Autodesk Inventor part; units mm, degrees
ref_plane "YZ Plane" through (0, 0, 0) normal (1, 0, 0) x (0, 1, 0)
ref_plane "XZ Plane" through (0, 0, 0) normal (0, 1, 0) x (-1, 0, 0)
ref_plane "XY Plane" through (0, 0, 0) normal (0, 0, 1) x (1, 0, 0)
sketch "Sketch1" plane through (0, 0, 0) normal (0, 0, 1) x (1, 0, 0)
  line L0 (9.6801, -14.008) -> (7.2052, -11.5331) construction
  line L1 (7.2052, -11.5331) -> (11.5893, -7.1491) construction
  line L2 (11.5893, -7.1491) -> (14.0642, -9.6239) construction
  line L3 (14.0642, -9.6239) -> (9.6801, -14.008) construction
  arc A0 (12.6369, -4.7496) -> (4.7496, -12.6369) centre (0, 0) ccw construction
  line L4 (10.9298, -3.0424) -> (12.6369, -4.7496) construction
  line L5 (11.6618, -4.6122) -> (10.9298, -3.0424) construction
  arc A1 (11.6618, -4.6122) -> (10.8551, -4.47) centre (11.2086, -4.8235) ccw construction
  line L6 (10.7915, -4.5335) -> (10.8551, -4.47) construction
  arc A2 (10.7915, -4.5335) -> (10.6527, -4.9738) centre (11.1451, -4.887) ccw construction
  line L7 (10.915, -6.4612) -> (10.6527, -4.9738) construction
  arc A3 (10.7761, -6.9016) -> (10.915, -6.4612) centre (10.4226, -6.548) ccw construction
  line L8 (6.9016, -10.7761) -> (10.7761, -6.9016) construction
  arc A4 (6.4612, -10.915) -> (6.9016, -10.7761) centre (6.548, -10.4226) ccw construction
  line L9 (6.4612, -10.915) -> (4.9738, -10.6527) construction
  arc A5 (4.9738, -10.6527) -> (4.5335, -10.7915) centre (4.887, -11.1451) ccw construction
  line L10 (4.5335, -10.7915) -> (4.47, -10.8551) construction
  arc A6 (4.47, -10.8551) -> (4.6122, -11.6618) centre (4.8235, -11.2086) ccw construction
  line L11 (4.6122, -11.6618) -> (3.0424, -10.9298) construction
  line L12 (3.0424, -10.9298) -> (4.7496, -12.6369) construction
  line L13 (-1.7167, -14.6498) -> (-1.7167, -17.5) construction
  line L14 (-1.7167, -17.5) -> (1.7167, -17.5) construction
  line L15 (1.7167, -14.6498) -> (1.7167, -17.5) construction
  arc A7 (1.7167, -14.6498) -> (6.9595, -13.0049) centre (0, 0) ccw construction
  arc A8 (6.9595, -13.0049) -> (8.2728, -15.1789) centre (8.2994, -13.6792) ccw construction
  line L16 (8.2728, -15.1789) -> (7.6816, -15.1684) construction
  arc A9 (8.5249, -17.8901) -> (7.6816, -15.1684) centre (7.655, -16.6682) ccw construction
  line L17 (8.5249, -17.8901) -> (13.5161, -14.3366) construction
  line L18 (13.5161, -14.3366) -> (13.5161, -12.2823) construction
  line L19 (13.5161, -12.2823) -> (14.6168, -12.2823) construction
  line L20 (14.6168, -12.2823) -> (14.6168, -1.9776) construction
  arc A10 (14.6168, -1.9776) -> (1.7167, 14.6498) centre (0, 0) ccw construction
  line L21 (1.7167, 14.6498) -> (1.7167, 17.5) construction
  line L22 (-1.7167, 17.5) -> (1.7167, 17.5) construction
  line L23 (-1.7167, 14.6498) -> (-1.7167, 17.5) construction
  arc A11 (-1.7167, 14.6498) -> (-14.2817, -3.6872) centre (0, 0) ccw construction
  line L24 (-14.2817, -3.6872) -> (-15.4135, -5.7935) construction
  arc A12 (-15.4135, -5.7935) -> (-14.5984, -8.502) centre (-13.6517, -6.7402) ccw construction
  line L25 (-14.5984, -8.502) -> (-9.6326, -11.1703) construction
  arc A13 (-9.6326, -11.1703) -> (-1.7167, -14.6498) centre (0, 0) ccw construction
  line L26 (-24.6, 24.6) -> (25.2, -25.2) construction
  line L27 (25.2, 24.6) -> (-24.6, -25.2) construction
  arc A14 (-1.4283, 10.15) -> (-9.5043, -3.8381) centre (0, 0) ccw
  circle A15 centre (0, 0) radius 10.1 construction
  line L28 (-1.4283, 10.15) -> (1.4283, 10.15)
  line L29 (-8.076, -6.3119) -> (-9.5043, -3.8381)
  line L30 (9.5043, -3.8381) -> (8.076, -6.3119)
  arc A16 (1.4283, 10.15) -> (-1.4283, 10.15) centre (0, 0) ccw
  arc A17 (9.5043, -3.8381) -> (1.4283, 10.15) centre (0, 0) ccw
  arc A18 (8.076, -6.3119) -> (9.5043, -3.8381) centre (0, 0) ccw
  arc A19 (-8.076, -6.3119) -> (8.076, -6.3119) centre (0, 0) ccw
  arc A20 (-9.5043, -3.8381) -> (-8.076, -6.3119) centre (0, 0) ccw
  arc A21 (10.7786, -4.5205) -> (10.6704, -4.6789) centre (11.1451, -4.887) ccw construction
  line L31 (10.7786, -4.5205) -> (10.8421, -4.457) construction
  arc A22 (11.7261, -4.7937) -> (10.8421, -4.457) centre (11.2086, -4.8235) ccw construction
  line L32 (11.7261, -4.7937) -> (10.8691, -2.9558) construction
  line L33 (10.8691, -2.9558) -> (12.6297, -4.7164) construction
  line L34 (4.7164, -12.6297) -> (2.9558, -10.8691) construction
  line L35 (2.9558, -10.8691) -> (4.4463, -11.5641) construction
  arc A23 (4.457, -10.8421) -> (4.4463, -11.5641) centre (4.8235, -11.2086) ccw construction
  line L36 (4.457, -10.8421) -> (4.5223, -10.7767) construction
  arc A24 (4.977, -10.6346) -> (4.6789, -10.6704) centre (4.887, -11.1451) ccw
  arc A25 (4.6789, -10.6704) -> (4.5223, -10.7767) centre (4.887, -11.1451) ccw construction
  arc A26 (10.6704, -4.6789) -> (10.6346, -4.977) centre (11.1451, -4.887) ccw
  circle A27 centre (0, 0) radius 12.65
  dimension "d4" = 20.2
  dimension "d5" = 10.15
  dimension "d6" = 20.5
  dimension "d9" = 360
  dimension "d28" = 25.3
extrude "Extrusion1" add sketch "Sketch1" against normal blind 3
sketch "Sketch3" plane through (0, 0, -3) normal (0, 0, -1) x (-1, 0, 0)
  circle A0 centre (0, 0) radius 10.25
  circle A1 centre (0, 0) radius 9
  circle A2 centre (0, 0) radius 11.5312
  circle A3 centre (0, 0) radius 12.65
  dimension "d17" = 18
extrude "Extrusion3" add sketch "Sketch3" along normal blind 10 contours A0 | A2 | A3
sketch "Sketch4" plane through (0, -10.7054, 0) normal (1, 0, 0) x (0, 0, -1)
  line L0 (13, 19.7054) -> (13, 1.7054)
  line L1 (3, 1.7054) -> (3, 19.7054)
  circle A0 centre (11, 10.7054) radius 1.4
  circle A1 centre (5, 10.7054) radius 1.4
  dimension "d24" = 2.8
  dimension "d25" = 2.8
  dimension "d26" = 6
  dimension "d27" = 2
extrude "Extrusion4" cut sketch "Sketch4" against normal through all
properties part number "30_focus_inlet_objective_mount_v7"
Model file for the job. Use its own axes, mm. A direction names the side the tool comes from. Round coordinates to 2 decimals unless told otherwise and drop trailing zeros. Order: outer loops, then holes, each group sorted by start corner. A loop starts at its lowest first (then second) coordinate and runs counter-clockwise, first axis right, second up. Notation, with made-up numbers: (16.5, -9) -> (29.5, -9) arc R19 cw to (29.5, 0) -> close; hole circle Ø7 at (32, 70.5). An arc over 180 degrees is marked (long way). Use one line per item in the form item = value.
Item 1: Cut at B-B, the plane x = 0. Write the cut outline in (y, z).
Returned:
outline = (-12.65, -13) -> (-9, -13) -> (-9, -3) -> (-10.25, -3) -> (-10.25, 0) -> (-12.65, 0) -> close; (9, -13) -> (12.65, -13) -> (12.65, 0) -> (10.25, 0) -> (10.25, -3) -> (9, -3) -> close
Item 2: Drill centre lines: line 1 (Z direction, x = -11.05, y = 0); line 2 (Y direction, x = 0, z = -7.75); line 3 (Z direction, x = 6.5, y = -7.5). Where is each one in solid material? Low to high.
Returned:
line_1 = -13 to -12.4, -9.6 to -6.4, -3.6 to 0
line_2 = -12.65 to -9, 9 to 12.65
line_3 = -13 to -3
Item 3: Cut at D-D, the plane z = -7.75. Write the cut outline in (x, y).
Returned:
outline = circle Ø25.3 at (0, 0); hole circle Ø18 at (0, 0)
Item 4: Cut at A-A, the plane y = 0. Write the cut outline in (x, z).
Returned:
outline = (-12.65, -13) -> (-9, -13) -> (-9, -12.4) -> (-12.65, -12.4) -> close; (-12.65, -9.6) -> (-9, -9.6) -> (-9, -6.4) -> (-12.65, -6.4) -> close; (-12.65, -3.6) -> (-9, -3.6) -> (-9, -3) -> (-10.25, -3) -> (-10.25, 0) -> (-12.65, 0) -> close; (9, -13) -> (12.65, -13) -> (12.65, 0) -> (10.25, 0) -> (10.25, -3) -> (9, -3) -> close
Item 5: Cut at C-C, the plane y = 5.75. Write the cut outline in (x, z).
Returned:
outline = (-11.27, -13) -> (-6.92, -13) -> (-6.92, -3) -> (-8.49, -3) -> (-8.49, 0) -> (-11.27, 0) -> close; (6.92, -13) -> (11.27, -13) -> (11.27, 0) -> (8.49, 0) -> (8.49, -3) -> (6.92, -3) -> close
Item 6: Pull direction Y, two halves, no side cores. Call faces 1 (the face through (-10.74, 0.06, -9.6)), 2 (the face through (-3, 9, -13)): released by +Y, released by -Y, zero draft, split by the parting line, or undercut.
Returned:
face_1 = undercut
face_2 = zero draft
Item 7: Flat gauge pins, fed straight in: pin 1 Ø8 at (x, y) = (3.5, -1.5) entering from -Z; pin 2 Ø1.5 at (x, z) = (9, -10) entering from -Y; pin 3 Ø1.5 at (y, z) = (-8, -3.5) entering from -X; pin 4 Ø4 at (y, z) = (-3, -7) entering from +X. Where does each tip first touch, or does it go through?
Returned:
pin_1 = through
pin_2 = -9.59
pin_3 = -10.37
pin_4 = 12.61
Item 8: Tool access for faces 3 (the face through (-0.1, 10.4, 0)), 4 (the face through (-10.74, -0.54, -6.29)), 5 (the face through (-8.81, 5.24, -1.48)): list every direction of +Z, -Z, +X, -X, +Y, -Y with a clear straight run to the whole face (end or side of a thin tool).
Returned:
face_3 = +Z, +X, -X, +Y, -Y
face_4 = -X
face_5 = +Z
